from build123d import *
from build123d.topology import SkipClean

# Parameters (mm, degrees)
SKETCH_1_R          = 8
EXTRUDE_1_DEPTH     = 3
SKETCH_2_R          = 10
SKETCH_2_R_2        = 8
EXTRUDE_3_DEPTH     = 1
SKETCH_4_R          = 8
EXTRUDE_4_DEPTH     = 3
EXTRUDE_START       = 1
SKETCH_5_R          = 10
SKETCH_5_R_2        = 8
EXTRUDE_5_DEPTH     = 1
SKETCH_6_W          = 57
SKETCH_6_H          = 57
EXTRUDE_6_DEPTH     = 3
CUT_EXTRUDE_1_DEPTH = 5
SKETCH_10_R         = 8.25
SKETCH_10_R_2       = 7.25
EXTRUDE_7_DEPTH     = 2
SKETCH_11_W         = 32
SKETCH_11_H         = 37
CUT_EXTRUDE_2_DEPTH = 57
SKETCH_12_W         = 57
SKETCH_12_H         = 57
SKETCH_12_W_2       = 54
SKETCH_12_H_2       = 54
EXTRUDE_8_DEPTH     = 85


with BuildPart() as part:
    # Sketch 1 → Extrude 1 (new body)
    with BuildSketch(Plane.XY):
        with BuildLine():
            Line((-16, 0), (-16, 56))
            Line((-16, 56), (-28.5, 56))
            Line((-28.5, 56), (-28.5, 96))
            Line((-28.5, 96), (28.5, 96))
            Line((28.5, 96), (28.5, 56))
            Line((28.5, 56), (16, 56))
            Line((16, 56), (16, 0))
            ThreePointArc((16, 0), (0, -16), (-16, 0))
        make_face()
        Circle(SKETCH_1_R, mode=Mode.SUBTRACT)
    extrude(amount=EXTRUDE_1_DEPTH)

    # Sketch 2 → Extrude 3 (add)
    with BuildSketch(Plane.XY.offset(3)):
        Circle(SKETCH_2_R)
        Circle(SKETCH_2_R_2, mode=Mode.SUBTRACT)
    extrude(amount=EXTRUDE_3_DEPTH)



with BuildPart() as body_2:
    # Sketch 4 → Extrude 4 (new body)
    with BuildSketch(Plane.XY.offset(29)):
        with BuildLine():
            Line((-16, 0), (-16, 56))
            Line((-16, 56), (-28.5, 56))
            Line((-28.5, 56), (-28.5, 96))
            Line((-28.5, 96), (28.5, 96))
            Line((28.5, 96), (28.5, 56))
            Line((28.5, 56), (16, 56))
            Line((16, 56), (16, 0))
            ThreePointArc((16, 0), (0, -16), (-16, 0))
        make_face()
        Circle(SKETCH_4_R, mode=Mode.SUBTRACT)
    extrude(amount=EXTRUDE_4_DEPTH)

    # Sketch 5 → Extrude 5 (add)
    with BuildSketch(Plane(origin=(0, 0, 29), x_dir=(-1, 0, 0), z_dir=(0, 0, -1)).offset(EXTRUDE_START)):
        with Locations(Location((0, 0, 0), (0, 0, 180))):
            Circle(SKETCH_5_R)
        with Locations(Location((0, 0, 0), (0, 0, 180))):
            Circle(SKETCH_5_R_2, mode=Mode.SUBTRACT)
    extrude(amount=-EXTRUDE_5_DEPTH)


with BuildPart() as part_1:
    add(part.part)

    add(body_2.part)  # Extrude 6 merges body 2
    # Sketch 6 → Extrude 6 (add)
    with BuildSketch(Plane.XZ.offset(-56)):
        with Locations((0, 19)):
            Rectangle(SKETCH_6_W, SKETCH_6_H)
    extrude(amount=-EXTRUDE_6_DEPTH)

    # Sketch 9 → Cut-Extrude 1 (cut)
    with BuildSketch(Plane.XZ.offset(-56)):
        with BuildLine():
            ThreePointArc((5.126524164, 24.126524164), (0, 26.25), (-5.126524164, 24.126524164))
            Line((-5.126524164, 24.126524164), (0, 19))
            Line((0, 19), (5.126524164, 24.126524164))
        make_face()
        with BuildLine():
            Line((0, 19), (-5.126524164, 24.126524164))
            ThreePointArc((-5.126524164, 24.126524164), (-7.25, 19), (-5.126524164, 13.873475836))
            Line((-5.126524164, 13.873475836), (0, 19))
        make_face()
        with BuildLine():
            Line((5.126524164, 24.126524164), (0, 19))
            Line((0, 19), (5.126524164, 13.873475836))
            ThreePointArc((5.126524164, 13.873475836), (6.698126611, 16.225545115), (7.25, 19))
            ThreePointArc((7.25, 19), (6.698126611, 21.774454885), (5.126524164, 24.126524164))
        make_face()
        with BuildLine():
            Line((5.126524164, 13.873475836), (0, 19))
            Line((0, 19), (-5.126524164, 13.873475836))
            ThreePointArc((-5.126524164, 13.873475836), (0, 11.75), (5.126524164, 13.873475836))
        make_face()
    extrude(amount=-CUT_EXTRUDE_1_DEPTH, mode=Mode.SUBTRACT)

    # Sketch 10 → Extrude 7 (add)
    with SkipClean():  # the faces are left unmerged after this step: merging them gives an invalid solid
        with BuildSketch(Plane(origin=(0, 59, 0), x_dir=(1, 0, 0), z_dir=(0, 1, 0))):
            with Locations((0, -19)):
                Circle(SKETCH_10_R)
            with Locations((0, -19)):
                Circle(SKETCH_10_R_2, mode=Mode.SUBTRACT)
        extrude(amount=EXTRUDE_7_DEPTH)

    # Sketch 11 → Cut-Extrude 2 (cut)
    with BuildSketch(Plane.ZY.offset(28.5)):
        with Locations((16, 77.5)):
            Rectangle(SKETCH_11_W, SKETCH_11_H)
    extrude(amount=-CUT_EXTRUDE_2_DEPTH, mode=Mode.SUBTRACT)

    # Sketch 12 → Extrude 8 (add)
    with BuildSketch(Plane(origin=(0, 59, 0), x_dir=(1, 0, 0), z_dir=(0, 1, 0))):
        with Locations((0, -19)):
            Rectangle(SKETCH_12_W, SKETCH_12_H)
        with Locations((0, -19)):
            Rectangle(SKETCH_12_W_2, SKETCH_12_H_2, mode=Mode.SUBTRACT)
    extrude(amount=EXTRUDE_8_DEPTH)


solid = part_1.part
Build history of the part. All positions in model axes, mm. A direction names the side the tool comes from. Give positions to 0.01 mm unless a question says otherwise; leave off trailing zeros. Loops run counter-clockwise (first coordinate to the right, second up) from the corner with the lowest first, then second, coordinate; pieces in that order, holes last. Notation, with made-up numbers: (49.25, -7.75) - (61.25, -7.75) arc R26 ccw to (61.25, 30.25) - close; hole circle Ø7 at (-36, -14). An arc over 180 degrees is marked (long way). Write item = value, one per line. Start each with the question number.
1) Pull direction X, two halves, no side cores. Call faces 5 (the flat face through (-7, 56, 26)), 6 (the flat face through (0, 101, 46)), 7 (the cylindrical face through (-9.99, -0.44, 28.49)): +X half, -X half, draft (parallel to the pull), parting line (faces both ways), or undercut.
2) Probe probe 1 along X at (y, z) = (80, 32); probe 2 along Z at (x, y) = (-9.5, 16.5); probe 3 along Z at (x, y) = (26, 133). List the from-to ranges inside material, lowest first. Write a range as from..to.
3) Band-saw the part on B-B on z = 8. Give the cut face in (x, y).
4) Tool access for faces 1 (the flat face through (0, -8.2, 28)), 2 (the flat face through (-27, 101, 19)), 3 (the flat face through (16, 28, 30)), 4 (the flat face through (-16, 28, 1)): list every direction of +Z, -Z, +X, -X, +Y, -Y with a clear straight run to the whole face (end or side of a thin tool).
5) Band-saw the part on D-D on z = 16.5. Give the cut face in (x, y), plus the area to 3 significant figures.
6) Drop flat-ended pins along their axis: pin 1 Ø9.5 at (x, y) = (7.5, 19) entering from +Z; pin 2 Ø21 at (x, y) = (0, 0) entering from -Z; pin 3 Ø6 at (x, y) = (-2, -1.5) entering from -Z; pin 4 Ø3.5 at (y, z) = (16.5, 1.5) entering from +X. Give the stop position or say it passes through.
7) Band-saw the part on C-C on x = 0. Count the separate pieces of the cut face and the enclosed holes in it, plus the area to 4 significant figures.
8) Band-saw the part on A-A on y = 96.5. Give the cut face in (x, z).
Final values:
q1.face_5 = draft
q1.face_6 = undercut
q1.face_7 = parting line
q2.probe_1 = -28.5..-27, 27..28.5
q2.probe_2 = 0..3, 29..32
q2.probe_3 = -9.5..-8, 46..47.5
q3.outline = (-28.5, 56) - (28.5, 56) - (28.5, 144) - (27, 144) - (27, 59) - (-27, 59) - (-27, 144) - (-28.5, 144) - close
q4.face_1 = +X, -X, -Y
q4.face_2 = +Y
q4.face_3 = +Z, -Z, +X, -Y
q4.face_4 = +Z, -Z, -X, -Y
q5.outline = (-28.5, 56) - (-6.81, 56) - (-6.81, 59) - (-27, 59) - (-27, 144) - (-28.5, 144) - close; (6.81, 56) - (28.5, 56) - (28.5, 144) - (27, 144) - (27, 59) - (6.81, 59) - close
q5.area = 385 mm²
q6.pin_1 = 32
q6.pin_2 = 0
q6.pin_3 = through
q6.pin_4 = 16
q7.separate_pieces = 4
q7.enclosed_holes = 0
q7.area = 726.5 mm²
q8.outline = (-28.5, -9.5) - (28.5, -9.5) - (28.5, 47.5) - (-28.5, 47.5) - close; hole (-27, -8) - (27, -8) - (27, 46) - (-27, 46) - close
